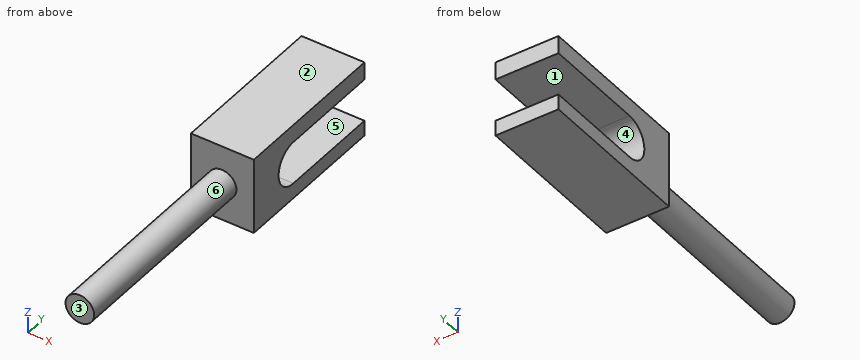
from build123d import *

# Parameters (mm, degrees)
SKETCH1_W           = 74.757250499
SKETCH1_H           = 56.340774555
BOSS_EXTRUDE1_DEPTH = 61.976
SKETCH2_R           = 21.051545166
CUT_EXTRUDE1_DEPTH  = 61.976
SKETCH3_W           = 61.976
SKETCH3_H           = 17.482215828
BOSS_EXTRUDE2_DEPTH = 101.6
SKETCH4_R           = 14.091408647
BOSS_EXTRUDE3_DEPTH = 203.2
SKETCH5_W           = 61.976
SKETCH5_H           = 15.17194434
BOSS_EXTRUDE4_DEPTH = 101.6


with BuildPart() as part:
    # Sketch1 → Boss-Extrude1 (new body)
    with BuildSketch(Plane(origin=(0, 0, 0), x_dir=(0, 0, -1), z_dir=(1, 0, 0))):
        with Locations((37.37862525, 28.170387278)):
            Rectangle(SKETCH1_W, SKETCH1_H)
    extrude(amount=BOSS_EXTRUDE1_DEPTH)

    # Sketch2 → Cut-Extrude1 (cut)
    with BuildSketch(Plane(origin=(61.976, 0, 0), x_dir=(0, 0, -1), z_dir=(1, 0, 0))):
        with Locations((38.533760994, 56.340774555)):
            Circle(SKETCH2_R)
    extrude(amount=-CUT_EXTRUDE1_DEPTH, mode=Mode.SUBTRACT)

    # Sketch3 → Boss-Extrude2 (add)
    with BuildSketch(Plane(origin=(0, 56.340774555, 0), x_dir=(1, 0, 0), z_dir=(0, 1, 0))):
        with Locations((30.988, 8.741107914)):
            Rectangle(SKETCH3_W, SKETCH3_H)
    extrude(amount=BOSS_EXTRUDE2_DEPTH)

    # Sketch4 → Boss-Extrude3 (add)
    with BuildSketch(Plane.XZ):
        with Locations(Location((30.69138806, -38.046002115, 0), (0, 0, 90))):
            Circle(SKETCH4_R)
    extrude(amount=BOSS_EXTRUDE3_DEPTH)

    # Sketch5 → Boss-Extrude4 (add)
    with BuildSketch(Plane(origin=(0, 56.340774555, 0), x_dir=(1, 0, 0), z_dir=(0, 1, 0))):
        with Locations((30.988, 67.171278329)):
            Rectangle(SKETCH5_W, SKETCH5_H)
    extrude(amount=BOSS_EXTRUDE4_DEPTH)


solid = part.part
The model under review builds one solid part; all positions refer to its coordinate system, in mm. Face numbers are marked on the shaded views. A direction names the side the tool comes from. Coordinates: 2 decimals unless noted, no trailing zeros. Write each loop counter-clockwise with the first axis right and the second up, starting at its lowest first coordinate (ties: lowest second). Pieces come first, ordered by that corner, then holes. Notation, with made-up numbers: (-36, -19) - (-17, -19) arc R30 ccw to (-17, 3) - close; hole circle Ø10 at (-10, -24). An arc over 180 degrees is marked (long way). Answer as a JSON object with one key per item and string values. Group by question number.
1. Add section D-D (y = -149). Give the boundary of the cut face in (x, z), plus the area to 3 significant figures.
2. Machinability: for the marked faces 1 and 2, which of the approach directions +Z, -Z, +X, -X, +Y, -Y give a long, thin tool a straight path to every point of the face, cutting with its end or side? Answer none if there is none.
3. Add section C-C (z = -46). Give the boundary of the cut face in (x, y).
4. Add section A-A (y = 84.5). Give the boundary of the cut face in (x, z).
5. Mouldability with a two-part tool opening along Z and no side actions: class the marked faces 3, 4, 5 and 6 as pulls with the +Z half, pulls with the -Z half, needs draft (parallel to the pull), parting line crosses it, or undercut.
6. Add section B-B (x = 7). Give the boundary of the cut face in (y, z), plus the area to 3 significant figures.
7. To check wall thickness, follow probe 1 along Z at (x, y) = (56, 79); probe 2 along Y at (x, z) = (19.5, -8.5); probe 3 along Z at (x, y) = (30.5, -48). State the ranges of each line that lie inside material, in increasing order.
8. Clearance check with flat-ended pins moving along their axes: pin 1 Ø3 at (y, z) = (-43, -29) entering from +X; pin 2 Ø8 at (x, z) = (14.5, -13.5) entering from -Y; pin 3 Ø8 at (y, z) = (-47.5, -56.5) entering from +X; pin 4 Ø6 at (y, z) = (-148.5, -33.5) entering from -X. State where each tip first meets the part, or that it passes through.
Findings:
{
 "1": {"outline": "circle Ø28.18 at (30.69, -38.05)", "area": "624 mm²"},
 "2": {"face 1": "+X, -X, +Y", "face 2": "+Z, +X, -X, +Y, -Y"},
 "3": {"outline": "(0, 0) - (19.06, 0) - (19.06, -203.2) - (42.32, -203.2) - (42.32, 0) - (61.98, 0) - (61.98, 36.66) - (0, 36.66) - close"},
 "4": {"outline": "(0, -74.76) - (61.98, -74.76) - (61.98, -59.59) - (0, -59.59) - close; (0, -17.48) - (61.98, -17.48) - (61.98, 0) - (0, 0) - close"},
 "5": {"face 3": "needs draft", "face 4": "undercut", "face 5": "undercut", "face 6": "parting line crosses it"},
 "6": {"outline": "(0, -74.76) - (157.94, -74.76) - (157.94, -59.59) - (56.34, -59.59) arc R21.05 cw to (56.34, -17.48) - (157.94, -17.48) - (157.94, 0) - (0, 0) - close", "area": "6,830 mm²"},
 "7": {"probe 1": "-74.76 to -59.59, -17.48 to 0", "probe 2": "0 to 157.94", "probe 3": "-52.14 to -23.96"},
 "8": {"pin 1": "x = 42.59", "pin 2": "y = 0", "pin 3": "through", "pin 4": "x = 16.69"}
}
